Could you check a few things on this model? Use its own coordinates, in mm. Coordinates: 2 decimals unless noted, no trailing zeros. Loops run counter-clockwise (first coordinate to the right, second up) from the corner with the lowest first, then second, coordinate; pieces in that order, holes last.
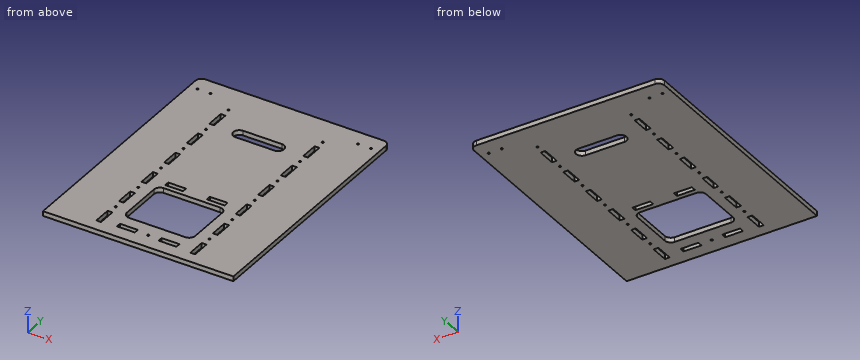
from build123d import *

# Parameters (mm, degrees)
SKETCH1_R           = 1.625
SKETCH1_R_2         = 1.65
SKETCH1_W           = 8
SKETCH1_H           = 30
SKETCH1_W_2         = 30
SKETCH1_H_2         = 8
BOSS_EXTRUDE1_DEPTH = 8
FILLET1_R           = 10
CUT_EXTRUDE1_DEPTH  = 9


with BuildPart() as part:
    # Sketch1 → Boss-Extrude1 (new body)
    with BuildSketch(Plane.XY):
        Polygon((0, 0), (320, 0), (320, 415), (160, 415), (0, 415), align=None)
        with Locations((14, 388)):
            Circle(SKETCH1_R, mode=Mode.SUBTRACT)
        with Locations((36, 388)):
            Circle(SKETCH1_R, mode=Mode.SUBTRACT)
        with Locations((284, 388)):
            Circle(SKETCH1_R, mode=Mode.SUBTRACT)
        with Locations((306, 388)):
            Circle(SKETCH1_R, mode=Mode.SUBTRACT)
        with Locations((81, 65)):
            Circle(SKETCH1_R_2, mode=Mode.SUBTRACT)
        with Locations((239, 65)):
            Circle(SKETCH1_R_2, mode=Mode.SUBTRACT)
        with Locations((81, 125)):
            Circle(SKETCH1_R_2, mode=Mode.SUBTRACT)
        with Locations((239, 125)):
            Circle(SKETCH1_R_2, mode=Mode.SUBTRACT)
        with Locations((81, 185)):
            Circle(SKETCH1_R_2, mode=Mode.SUBTRACT)
        with Locations((239, 185)):
            Circle(SKETCH1_R_2, mode=Mode.SUBTRACT)
        with Locations((81, 245)):
            Circle(SKETCH1_R_2, mode=Mode.SUBTRACT)
        with Locations((239, 245)):
            Circle(SKETCH1_R_2, mode=Mode.SUBTRACT)
        with Locations((81, 305)):
            Circle(SKETCH1_R_2, mode=Mode.SUBTRACT)
        with Locations((239, 305)):
            Circle(SKETCH1_R_2, mode=Mode.SUBTRACT)
        with Locations((81, 365)):
            Circle(SKETCH1_R_2, mode=Mode.SUBTRACT)
        with Locations((239, 365)):
            Circle(SKETCH1_R_2, mode=Mode.SUBTRACT)
        with Locations((160, 26.566938385)):
            Circle(SKETCH1_R_2, mode=Mode.SUBTRACT)
        with BuildLine():
            Line((112.646025267, 142.602367126), (207.353974733, 142.602367126))
            ThreePointArc((207.353974733, 142.602367126), (214.425042545, 139.673434938), (217.353974733, 132.602367126))
            Line((217.353974733, 132.602367126), (217.353974733, 60.566938385))
            ThreePointArc((217.353974733, 60.566938385), (214.425042545, 53.495870573), (207.353974733, 50.566938385))
            Line((207.353974733, 50.566938385), (112.646025267, 50.566938385))
            ThreePointArc((112.646025267, 50.566938385), (105.574957455, 53.495870573), (102.646025267, 60.566938385))
            Line((102.646025267, 60.566938385), (102.646025267, 132.602367126))
            ThreePointArc((102.646025267, 132.602367126), (105.574957455, 139.673434938), (112.646025267, 142.602367126))
        make_face(mode=Mode.SUBTRACT)
        with Locations((81, 35)):
            Rectangle(SKETCH1_W, SKETCH1_H, mode=Mode.SUBTRACT)
        with Locations((195, 26.566938385)):
            Rectangle(SKETCH1_W_2, SKETCH1_H_2, mode=Mode.SUBTRACT)
        with Locations((125, 26.566938385)):
            Rectangle(SKETCH1_W_2, SKETCH1_H_2, mode=Mode.SUBTRACT)
        with Locations((125, 154.566938385)):
            Rectangle(SKETCH1_W_2, SKETCH1_H_2, mode=Mode.SUBTRACT)
        with Locations((195, 154.566938385)):
            Rectangle(SKETCH1_W_2, SKETCH1_H_2, mode=Mode.SUBTRACT)
        with Locations((239, 35)):
            Rectangle(SKETCH1_W, SKETCH1_H, mode=Mode.SUBTRACT)
        with Locations((81, 95)):
            Rectangle(SKETCH1_W, SKETCH1_H, mode=Mode.SUBTRACT)
        with Locations((239, 95)):
            Rectangle(SKETCH1_W, SKETCH1_H, mode=Mode.SUBTRACT)
        with Locations((81, 155)):
            Rectangle(SKETCH1_W, SKETCH1_H, mode=Mode.SUBTRACT)
        with Locations((239, 155)):
            Rectangle(SKETCH1_W, SKETCH1_H, mode=Mode.SUBTRACT)
        with Locations((81, 215)):
            Rectangle(SKETCH1_W, SKETCH1_H, mode=Mode.SUBTRACT)
        with Locations((239, 215)):
            Rectangle(SKETCH1_W, SKETCH1_H, mode=Mode.SUBTRACT)
        with Locations((81, 275)):
            Rectangle(SKETCH1_W, SKETCH1_H, mode=Mode.SUBTRACT)
        with Locations((239, 275)):
            Rectangle(SKETCH1_W, SKETCH1_H, mode=Mode.SUBTRACT)
        with Locations((81, 335)):
            Rectangle(SKETCH1_W, SKETCH1_H, mode=Mode.SUBTRACT)
        with Locations((239, 335)):
            Rectangle(SKETCH1_W, SKETCH1_H, mode=Mode.SUBTRACT)
    extrude(amount=BOSS_EXTRUDE1_DEPTH)

    # Fillet1
    fillet1_edges = [part.edges().sort_by_distance(p)[0] for p in [
        (0, 415, 4),
        (320, 415, 4),
    ]]
    fillet(fillet1_edges, radius=FILLET1_R)

    # Sketch2 → Cut-Extrude1 (cut, through all)
    with BuildSketch(Plane(origin=(0, 0, 0), x_dir=(-1, 0, 0), z_dir=(0, 0, -1))):
        with BuildLine():
            Line((-192.5, 330), (-127.5, 330))
            ThreePointArc((-127.5, 330), (-117.5, 320), (-127.5, 310))
            Line((-127.5, 310), (-192.5, 310))
            ThreePointArc((-192.5, 310), (-202.5, 320), (-192.5, 330))
        make_face()
    extrude(amount=-CUT_EXTRUDE1_DEPTH, mode=Mode.SUBTRACT)


solid = part.part
(1) I need wall thicknesses on probe 1 along X at (y, z) = (65, 2.5); probe 2 along X at (y, z) = (228.5, 2.5); probe 3 along X at (y, z) = (388, 5.5) (3 decimals). Which ranges of each line are inside material? Lowest first, please.
Answers:
probe 1: x = 0 to 79.35, 82.65 to 102.65, 217.35 to 237.35, 240.65 to 320
probe 2: x = 0 to 77, 85 to 235, 243 to 320
probe 3: x = 0 to 12.375, 15.625 to 34.375, 37.625 to 282.375, 285.625 to 304.375, 307.625 to 320
(2) Imagine slicing it at B-B, the plane y = 104. Write out the boundary of the cut face in (x, z), and give its area (3 significant figures).
Answers:
outline: (0, 0) - (77, 0) - (77, 8) - (0, 8) - close; (85, 0) - (102.65, 0) - (102.65, 8) - (85, 8) - close; (217.35, 0) - (235, 0) - (235, 8) - (217.35, 8) - close; (243, 0) - (320, 0) - (320, 8) - (243, 8) - close
area: 1,510 mm2
(3) Imagine slicing it at A-A, the plane y = 281.5. Write out the boundary of the cut face in (x, z).
Answers:
outline: (0, 0) - (77, 0) - (77, 8) - (0, 8) - close; (85, 0) - (235, 0) - (235, 8) - (85, 8) - close; (243, 0) - (320, 0) - (320, 8) - (243, 8) - close
(4) Imagine slicing it at C-C, the plane z = 3. State how many separate pieces and enclosed holes the cut face has, and give its area (3 significant figures).
Answers:
separate pieces: 1
enclosed holes: 35
area: 117,000 mm2
